from build123d import *

# Parameters (mm, degrees)
SKETCH005_W             = 58
SKETCH005_H             = 20
SKETCH005_R             = 2.75
PAD004_DEPTH            = 8
SKETCH006_R             = 2.25
PAD005_DEPTH            = 4
POCKET005_DEPTH         = 4
SKETCH011_W             = 15
SKETCH011_H             = 2.666667
POCKET007_DEPTH         = 20
SKETCH012_W             = 18
SKETCH012_H             = 4
POCKET008_DEPTH         = 8
FILLET_R                = 0.5
BODY002_PLACEMENT_ANGLE = 180


with BuildPart() as part:
    # Sketch005 → Pad004 (new body)
    with BuildSketch(Plane.XZ):
        Rectangle(SKETCH005_W, SKETCH005_H)
        with Locations((0, 2)):
            Circle(SKETCH005_R, mode=Mode.SUBTRACT)
    extrude(amount=PAD004_DEPTH)

    # Sketch006 (on Face4 of Pad004) → Pad005 (join)
    with BuildSketch(Plane(origin=(-29, 0, 0), x_dir=(0, 0, -1), z_dir=(-1, 0, 0))):
        with BuildLine():
            Line((-10, 0), (10, 0))
            Line((10, 0), (10, 35.5))
            ThreePointArc((10, 35.5), (0, 45.5), (-10, 35.5))
            Line((-10, 35.5), (-10, 0))
        make_face()
        with Locations((0, 40)):
            Circle(SKETCH006_R, mode=Mode.SUBTRACT)
    pad005 = extrude(amount=PAD005_DEPTH)

    # Mirrored003: Pad005 across YZ
    add(pad005.mirror(Plane.YZ))

    # Sketch007 (on Face5 of Mirrored003) → Pocket005 (cut)
    with BuildSketch(Plane.XZ.offset(8)):
        Polygon((4.113621, 4.375), (0, 6.75), (-4.113621, 4.375), (-4.113621, -0.375), (0, -2.75), (4.113621, -0.375), align=None)
    extrude(amount=-POCKET005_DEPTH, mode=Mode.SUBTRACT)

    # Sketch011 (on Face14 of Pocket005) → Pocket007 (cut)
    with BuildSketch(Plane(origin=(0, 0, 10), x_dir=(-1, 0, 0), z_dir=(0, 0, 1))):
        with Locations((-19.5, 4.169504)):
            Rectangle(SKETCH011_W, SKETCH011_H)
    pocket007 = extrude(amount=-POCKET007_DEPTH, mode=Mode.SUBTRACT)

    # Mirrored004: Pocket007 across YZ
    add(pocket007.mirror(Plane.YZ), mode=Mode.SUBTRACT)

    # Sketch012 (on Face3 of Mirrored004) → Pocket008 (cut)
    with BuildSketch(Plane(origin=(0, 0, 0), x_dir=(1, 0, 0), z_dir=(0, 1, 0))):
        with Locations((0, 8)):
            Rectangle(SKETCH012_W, SKETCH012_H)
    extrude(amount=-POCKET008_DEPTH, mode=Mode.SUBTRACT)

    # Fillet
    fillet_edges = [part.edges().sort_by_distance(p)[0] for p in [
        (0, -8, -6),
        (9, -8, -8),
        (-9, -8, -8),
    ]]
    fillet(fillet_edges, radius=FILLET_R)


with BuildPart() as part_1:
    # Body002 placement: moved
    add(part.part.moved(Location((0, -15, -23))).rotate(Axis((0, -15, -23), (1, 0, 0)), BODY002_PLACEMENT_ANGLE))


solid = part_1.part
Check sheet for the modelled part. Datum: model origin and axes. Units: mm. A direction names the side the tool comes from. Give positions to 0.01 mm unless a question says otherwise; leave off trailing zeros. Loops run counter-clockwise (first coordinate to the right, second up) from the corner with the lowest first, then second, coordinate; pieces in that order, holes last. Notation, with made-up numbers: M 87,0 L 115,0 A23 cw 115,35 Z; hole C -4.75,33.5 d6. An arc over 180 degrees is marked long. Use a Markdown table: item, result. Add a question column.
Q1. Scan lines: line 1 along X through (y, z) = (-1, -20.25); line 2 along Z through (x, y) = (0, -13); line 3 along Y through (x, z) = (-26, -25.75). Record each from-to range of solid material in increasing order. Write a range as [from, to].
Q2. Tool access check on faces 4 (the flat face through (9, -11, -15)), 5 (the flat face through (-4.114, -9, -25)), 6 (the flat face through (-12, -11, -23)). Record the directions out of +Z, -Z, +X, -X, +Y, -Y that give a thin tool (end or side, any length) a straight path to the whole face; none if there is none.
Q3. Sectioned sample at B-B, the plane z = -15. Record the cut outline in (x, y).
Q4. Go/stop test with flat-tipped pins: pin 1 (6 mm diameter, centred on x = 8.5, z = -21.5, fed in from +Y); pin 2 (2.5 mm diameter, centred on y = 25, z = -23, fed in from -X). Record where each tip stops, or that it passes through.
Q5. Sectioned sample at D-D, the plane x = -5. Record the cut outline in (y, z).
Q6. Sectioned sample at C-C, the plane x = -16.5. Record the cut outline in (y, z), then the cut area to 3 significant figures.
Q7. Sectioned sample at A-A, the plane y = -3. Record the cut outline in (x, z), then the cut area to 3 significant figures.
Q8. Mould release check, pull along Z, two halves, no side actions. Record for faces 1 (the flat face through (25, -8, -13)), 2 (the flat face through (4.114, -9, -25)), 3 (the cylindrical face through (-31, 30.5, -22.8)): pulls with the +Z half, pulls with the -Z half, needs draft (parallel to the pull), parting line crosses it, or undercut.
Verdict:
| question | item | result |
|---|---|---|
| 1 | line 1 | [-33, -29], [29, 33] |
| 1 | line 2 | [-33, -27.75], [-22.25, -17] |
| 1 | line 3 | [-15, -12.16], [-9.5, -7] |
| 2 | face 4 | +Z, +Y, -Y |
| 2 | face 5 | +Y |
| 2 | face 6 | +Z, -Z |
| 3 | outline | M -33,-15 L -9,-15 L -9,-7.5 A0.5 ccw -9.5,-7 L -29,-7 L -29,26.5 L -33,26.5 Z; M 9,-15 L 33,-15 L 33,26.5 L 29,26.5 L 29,-7 L 9.5,-7 A0.5 ccw 9,-7.5 Z; hole M -27,-12.16 L -12,-12.16 L -12,-9.5 L -27,-9.5 Z; hole M 12,-12.16 L 27,-12.16 L 27,-9.5 L 12,-9.5 Z |
| 4 | pin 1 | y = -7 |
| 4 | pin 2 | through |
| 5 | outline | M -15,-33 L -7,-33 L -7,-17.5 A0.5 ccw -7.5,-17 L -15,-17 Z |
| 6 | outline | M -15,-33 L -12.16,-33 L -12.16,-13 L -15,-13 Z; M -9.5,-33 L -7,-33 L -7,-13 L -9.5,-13 Z |
| 6 | area | 107 mm^2 |
| 7 | outline | M -33,-33 L -29,-33 L -29,-13 L -33,-13 Z; M 29,-33 L 33,-33 L 33,-13 L 29,-13 Z |
| 7 | area | 160 mm^2 |
| 8 | face 1 | pulls with the +Z half |
| 8 | face 2 | undercut |
| 8 | face 3 | parting line crosses it |
